```python
from build123d import *

# Parameters (mm, degrees)
SKETCH_1_R      = 16
SKETCH_1_R_2    = 12.5
EXTRUDE_1_DEPTH = 35
SKETCH_2_R      = 16
SKETCH_2_R_2    = 12.5
EXTRUDE_2_DEPTH = 35
SKETCH_4_R      = 16
SKETCH_4_R_2    = 12.5
EXTRUDE_3_DEPTH = 35
REVOLVE_1_ANGLE = 90


with BuildPart() as part:
    # 草图1 → 凸台-拉伸1 (new body)
    with BuildSketch(Plane.XY):
        Circle(SKETCH_1_R)
        Circle(SKETCH_1_R_2, mode=Mode.SUBTRACT)
    extrude(amount=EXTRUDE_1_DEPTH)

    # 草图2 → 凸台-拉伸2 (add)
    with BuildSketch(Plane(origin=(0, 0, 0), x_dir=(0, 0, -1), z_dir=(1, 0, 0))):
        Circle(SKETCH_2_R)
        Circle(SKETCH_2_R_2, mode=Mode.SUBTRACT)
    extrude(amount=EXTRUDE_2_DEPTH)

    # 草图4 → 凸台-拉伸3 (add)
    with BuildSketch(Plane(origin=(0, 0, 0), x_dir=(1, 0, 0), z_dir=(0, 1, 0))):
        Circle(SKETCH_4_R)
        Circle(SKETCH_4_R_2, mode=Mode.SUBTRACT)
    extrude(amount=EXTRUDE_3_DEPTH)

    # 草图3 → 旋转1 (revolve)
    with BuildSketch(Plane.XY):
        with BuildLine():
            Line((0, 16), (0, -16))
            ThreePointArc((0, -16), (-16, 0), (0, 16))
        make_face()
    revolve(axis=Axis((0, 16, 0), (0, -1, 0)), revolution_arc=REVOLVE_1_ANGLE)


solid = part.part
```
The model under review builds one solid part; all positions refer to its coordinate system, in mm. A direction names the side the tool comes from. Round coordinates to 2 decimals unless told otherwise and drop trailing zeros. Loops run counter-clockwise (first coordinate to the right, second up) from the corner with the lowest first, then second, coordinate; pieces in that order, holes last.
1) Consider section A-A on x = -6. State the section outline as (y, z) points.
Values follow:
outline: (-14.83, 0) arc R14.83 ccw to (0, -14.83) - (35, -14.83) - (35, -10.97) - (9.99, -10.97) arc R14.83 ccw to (14.83, 0) - (14.83, 10.97) - (35, 10.97) - (35, 14.83) - (14.83, 14.83) - (14.83, 35) - (10.97, 35) - (10.97, 14.83) - (0, 14.83) - (0, 10.97) - (10.97, 10.97) - (10.97, 0) - (-10.97, 0) - (-10.97, 35) - (-14.83, 35) - close
2) Tool access review of faces 1 (the face through (-9.92, -7.606, 21.144)), 2 (the face through (12, 0, -7)), 3 (the face through (9, 10, 0)), 4 (the face through (-10, 35, 8)): name each direction out of +Z, -Z, +X, -X, +Y, -Y from which nothing blocks a thin tool from reaching the whole face with its end or side.
Values follow:
face 1: +Z
face 2: +X
face 3: none
face 4: +Z, -Z, +X, -X, +Y
3) Consider section B-B on y = 25.5. State the section outline as (x, z) points, then the cut area to 3 significant figures.
Values follow:
outline: circle Ø32 at (0, 0); hole circle Ø25 at (0, 0)
area: 313 mm2
4) Consider section C-C on z = -1. State the section outline as (x, y) points, then the cut area to 3 significant figures.
Values follow:
outline: (-15.97, 0) arc R15.97 ccw to (0, -15.97) - (35, -15.97) - (35, -12.46) - (0, -12.46) - (0, 12.46) - (12.46, 12.46) - (12.46, 0) - (15.97, 0) - (15.97, 12.46) - (35, 12.46) - (35, 15.97) - (15.97, 15.97) - (15.97, 35) - (12.46, 35) - (12.46, 15.97) - (0, 15.97) arc R15.97 ccw to (-12.46, 9.99) - (-12.46, 35) - (-15.97, 35) - close
area: 856 mm2
5) Wall thickness on line 1 along Z through (x, y) = (18.5, 0.5); line 2 along Y through (x, z) = (28.5, 0): over which ranges is each line inside the solid? List them lowest first.
Values follow:
line 1: z = -15.99 to -12.49, 12.49 to 15.99
line 2: y = -16 to -12.5, 12.5 to 16
6) The part is to be moulded in two halves that separate along Y. For faces 5 (the face through (21.144, -14.195, -7.383)), 6 (the face through (-10, -8, 35)), 7 (the face through (0, 10, 10)), say which applies: pulls with the +Y half, pulls with the -Y half, needs draft (parallel to the pull), parting line crosses it, or undercut.
Values follow:
face 5: parting line crosses it
face 6: needs draft
face 7: undercut
7) Clearance check with flat-ended pins moving along their axes: P1, Ø10, axis at x = 7.5, z = 7.5, coming from the -Y side; P2, Ø4, axis at x = -4, y = -6, coming from the +Z side; P3, Ø8, axis at y = 12, z = 8.5, coming from the -X side. State where each tip first meets the part, or that it passes through.
Values follow:
P1: stops at y = -15.8
P2: stops at z = 0
P3: stops at x = -15.35
